CAD build for the part. Positions are in the model's coordinates, mm. Face numbers are marked on the shaded views. Round coordinates to 2 decimals unless told otherwise and drop trailing zeros. Order: outer loops, then holes, each group sorted by start corner. A loop starts at its lowest first (then second) coordinate and runs counter-clockwise, first axis right, second up. Notation, with made-up numbers: (0.25, -1) -> (54.25, -1) arc R17 ccw to (54.25, 22) -> close; hole circle Ø5 at (81.5, 66). An arc over 180 degrees is marked (long way). Return JSON: item names as keys, results as strings. Group by question number.
Q1. Probe line 1 along Z through (x, y) = (0.35, -0.5); line 2 along Y through (x, z) = (0.5, 7.75); line 3 along Y through (x, z) = (-0.85, 6.75). List the from-to ranges inside material, lowest first.
Q2. Mould opens along Z. For the marked faces 1, 2 and 3 say: +Z half, -Z half, draft (parallel to the pull), parting line (faces both ways), or undercut.
Q3. Flat gauge pin, fed straight in: pin 1 (1.5 mm diameter, centred on x = 0.5, y = -1.5, fed in from +Z). Where does the tip first touch, or does it go through?
Q4. Cut at A-A (z = 2.75). Write the cut outline in (x, y), then the cut area to 3 significant figures.
Q5. Cut at D-D (y = -5.25). Write the cut outline in (x, z), then the cut area to 3 significant figures.
Q6. Cut at B-B (x = 0.9). Write the cut outline in (y, z), then the cut area to 3 significant figures.
Q7. Cut at C-C (y = -0.25). Write the cut outline in (x, z), then the cut area to 3 significant figures.
from build123d import *

# Parameters (mm, degrees)
F1_DEPTH     = 1.27
F2_W         = 1.8970449455
F2_H         = 3.5115340725
F3_DEPTH     = 1.016
F4_T4_DEPTH  = 1.8970449455
F4_T9_DEPTH  = 3.5115340725
F4_T14_DEPTH = 1.8970449455
F4_T19_DEPTH = 3.5115340725


# Not quite as in the source:
# - a fillet or chamfer that OpenCascade refuses, or shapes differently, is made with other operations: its cross-section is extruded or revolved along the edge and cut away or added


with BuildPart() as f1:
    # F0 (on Right) → F1 (new body, symmetric)
    with BuildSketch(Plane.YZ):
        Polygon((-5.8383567513, 4.1238272734), (-6.2, 4.1238272734), (-6.2, 0), (0, 0), (0, 5.1), (-0.7954361361, 5.1), (-1.9601408858, 8.3), (-4.3183541857, 8.3), align=None)
    extrude(amount=F1_DEPTH, both=True)

    # F2 (on face) → F3 (cut)
    with BuildSketch(Plane(origin=(0, 0, 0), x_dir=(-1, 0, 0), z_dir=(0, 1, 0))):
        with Locations((0, 2.7114218101)):
            Rectangle(F2_W, F2_H)
    extrude(amount=-F3_DEPTH, mode=Mode.SUBTRACT)

    # F4: chamfer of 5.08 x 0.895741062 on 4 edges, made by hand


with BuildPart() as f4_tool2:
    # F4_s3 → F4_t4 (new body)
    with BuildSketch(Plane.YZ.offset(-0.9485224728)):
        Polygon((4.064, 4.4671888463), (-1.016, 3.5714477843), (-1.016, 4.4671888463), align=None)
    extrude(amount=F4_T4_DEPTH)

    split(bisect_by=Plane.XZ, keep=Keep.TOP)


with BuildPart() as f1_1:
    add(f1.part)

    # F4_t1: union F4_tool2
    add(f4_tool2.part)


with BuildPart() as f4_tool7:
    # F4_s8 → F4_t9 (new body)
    with BuildSketch(Plane.XY.offset(4.4671888463)):
        Polygon((0.9485224728, 4.064), (0.0527814108, -1.016), (0.9485224728, -1.016), align=None)
    extrude(amount=-F4_T9_DEPTH)

    split(bisect_by=Plane.XZ, keep=Keep.TOP)


with BuildPart() as f1_2:
    add(f1_1.part)

    # F4_t6: union F4_tool7
    add(f4_tool7.part)


with BuildPart() as f4_tool12:
    # F4_s13 → F4_t14 (new body)
    with BuildSketch(Plane.YZ.offset(0.9485224728)):
        Polygon((4.064, 0.9556547739), (-1.016, 1.8513958359), (-1.016, 0.9556547739), align=None)
    extrude(amount=-F4_T14_DEPTH)

    split(bisect_by=Plane.XZ, keep=Keep.TOP)


with BuildPart() as f1_3:
    add(f1_2.part)

    # F4_t11: union F4_tool12
    add(f4_tool12.part)


with BuildPart() as f4_tool17:
    # F4_s18 → F4_t19 (new body)
    with BuildSketch(Plane.XY.offset(0.9556547739)):
        Polygon((-0.9485224728, 4.064), (-0.0527814108, -1.016), (-0.9485224728, -1.016), align=None)
    extrude(amount=F4_T19_DEPTH)

    split(bisect_by=Plane.XZ, keep=Keep.TOP)


with BuildPart() as f1_4:
    add(f1_3.part)

    # F4_t16: union F4_tool17
    add(f4_tool17.part)


solid = f1_4.part
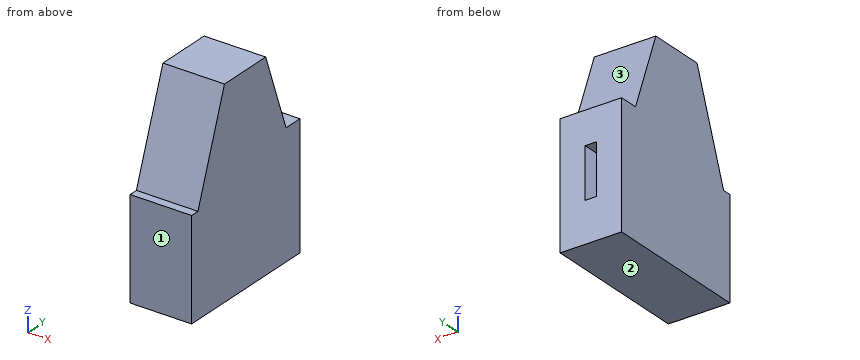
Solution:
{
 "1": {"line 1": "z = 0 to 5.1", "line 2": "y = -4.52 to -1.76", "line 3": "y = -4.88 to -1.4"},
 "2": {"face 1": "draft", "face 2": "-Z half", "face 3": "+Z half"},
 "3": {"pin 1": "stops at z = 8.3"},
 "4": {"outline": "(-1.27, -6.2) -> (1.27, -6.2) -> (1.27, 0) -> (0.23, 0) -> (0.05, -1.02) -> (-0.05, -1.02) -> (-0.23, 0) -> (-1.27, 0) -> close", "area": "15.5 mm²"},
 "5": {"outline": "(-1.27, 0) -> (1.27, 0) -> (1.27, 5.74) -> (-1.27, 5.74) -> close", "area": "14.6 mm²"},
 "6": {"outline": "(-6.2, 0) -> (0, 0) -> (0, 5.1) -> (-0.8, 5.1) -> (-1.96, 8.3) -> (-4.32, 8.3) -> (-5.84, 4.12) -> (-6.2, 4.12) -> close", "area": "42.4 mm²"},
 "7": {"outline": "(-1.27, 0) -> (1.27, 0) -> (1.27, 5.1) -> (-1.27, 5.1) -> close; hole (-0.19, 1.72) -> (0.19, 1.72) -> (0.19, 3.71) -> (-0.19, 3.71) -> close", "area": "12.2 mm²"}
}
